```python
from build123d import *
from OCP.BRepFilletAPI import BRepFilletAPI_MakeChamfer

# Parameters (mm, degrees)
BOSS_EXTRUDE1_DEPTH     = 2.4
CUT_EXTRUDE1_DEPTH      = 15.66535032
CUT_EXTRUDE1_DEPTH_BACK = 2.1
SKETCH4_R               = 0.55
CUT_EXTRUDE2_START      = -9
CUT_EXTRUDE2_DEPTH      = 9
SKETCH6_W               = 4.2
SKETCH6_H               = 1.75
BOSS_EXTRUDE2_DEPTH     = 0.75
BOSS_EXTRUDE3_DEPTH     = 0.5
FILLET1_R               = 1
FILLET2_R               = 2
FILLET3_R               = 1
FILLET4_R               = 2
FILLET6_R               = 0.5
FILLET8_R               = 0.6
FILLET9_R               = 3
FILLET10_R              = 3
CHAMFER1_SIZE           = 0.3
CHAMFER1_SIZE2          = 0.357526078


# Read off the part's stored shape, not the designer's step: Cut-Extrude2
# Some blends are built 0.0001 mm under size
with BuildPart() as part:
    # Sketch1 → Boss-Extrude1 (new body)
    with BuildSketch(Plane(origin=(0, 0, 0), x_dir=(1, 0, 0), z_dir=(0, 1, 0))):
        Polygon((-2.1, 0), (-2.1, 5.75), (-1.1, 5.75), (-1.1, 7.25), (-2.1, 7.25), (-4.1, 7.25), (-4.1, 1), (-6.55, -1), (-6.55, -5.65), (-4.05, -5.65), (-4.05, -1.75), (4.05, -1.75), (4.05, -5.65), (6.55, -5.65), (6.55, -1), (4.1, 1), (4.1, 7.25), (2.1, 7.25), (1.1, 7.25), (1.1, 5.75), (2.1, 5.75), (2.1, 0), align=None)
    extrude(amount=BOSS_EXTRUDE1_DEPTH)

    # Sketch4 → Cut-Extrude1 (cut, two sides: drawn at the far end of the back side and taken through both)
    with BuildSketch(Plane.XY.offset(5.65).offset(-CUT_EXTRUDE1_DEPTH_BACK)):
        with Locations((-5.3, 1.2)):
            Circle(SKETCH4_R)
        with Locations(Location((5.3, 1.2, 0), (0, 0, 180))):
            Circle(SKETCH4_R)
    extrude(amount=CUT_EXTRUDE1_DEPTH + CUT_EXTRUDE1_DEPTH_BACK, mode=Mode.SUBTRACT)

    # Cut-Extrude2 outline → Cut-Extrude2 (cut)
    with BuildSketch(Plane.XY.offset(1.75).offset(CUT_EXTRUDE2_START)):
        Polygon((-1.700147862, 2.4), (0, 0.699852138), (1.700147862, 2.4), align=None)
    extrude(amount=CUT_EXTRUDE2_DEPTH, mode=Mode.SUBTRACT)

    # Sketch6 → Boss-Extrude2 (add)
    with BuildSketch(Plane.XZ):
        with Locations((0, 0.875)):
            Rectangle(SKETCH6_W, SKETCH6_H)
    extrude(amount=BOSS_EXTRUDE2_DEPTH)

    # Sketch7 → Boss-Extrude3 (add)
    with BuildSketch(Plane.XZ):
        Polygon((-2.1, -5.75), (-1.1, -5.75), (-1.1, -7.25), (-4.1, -7.25), (-4.1, -2), (-2.1, -2), align=None)
        Polygon((4.1, -2), (2.1, -2), (2.1, -5.75), (1.1, -5.75), (1.1, -7.25), (4.1, -7.25), align=None)
    extrude(amount=BOSS_EXTRUDE3_DEPTH)

    # Fillet1
    # the kernel refuses this fillet: 1 mm, written as the material it adds along each edge
    with BuildSketch(Plane(origin=(-2.1, 0, 1.75), x_dir=(-1, 0, 0), z_dir=(0, 0, -1))) as fillet1_piece_1:
        with BuildLine():
            CenterArc((0.968245837, -1), FILLET1_R, 90, 75.522487814)
            Line((0, -0.75), (0, 0))
            Line((0, 0), (0.968245837, 0))
        make_face()
    extrude(amount=1.75)
    with BuildSketch(Plane(origin=(2.1, 0, 0), x_dir=(0, -1, 0), z_dir=(0, 0, 1))) as fillet1_piece_2:
        with BuildLine():
            CenterArc((1, 0.968245837), FILLET1_R, 180, 75.522487814)
            Line((0, 0.968245837), (0, 0))
            Line((0, 0), (0.75, 0))
        make_face()
    extrude(amount=1.75)

    # Fillet2
    fillet2_edges = [part.edges().sort_by_distance(p)[0] for p in [
        (-2.1, -0.75, 0.875),
        (2.1, -0.75, 0.875),
    ]]
    fillet(fillet2_edges, radius=FILLET2_R)

    # Fillet3
    fillet3_edges = [part.edges().sort_by_distance(p)[0] for p in [
        (-2.1, 0.95, -5.75),
        (2.1, 0.95, -5.75),
        (-2.1, 1.2, 0),
        (2.1, 1.2, 0),
    ]]
    fillet(fillet3_edges, radius=FILLET3_R - 0.0001)  # a hair under: the kernel refuses the full size

    # Fillet4
    fillet4_edges = [part.edges().sort_by_distance(p)[0] for p in [
        (-4.1, 0.95, -7.25),
        (4.1, 0.95, -7.25),
    ]]
    fillet(fillet4_edges, radius=FILLET4_R)

    # Fillet6
    fillet6_edges = [part.edges().sort_by_distance(p)[0] for p in [
        (-1.1, 0.649926069, -7.25),
        (1.1, 0.649926069, -7.25),
    ]]
    fillet(fillet6_edges, radius=FILLET6_R)

    # Fillet8
    fillet8_edges = [part.edges().sort_by_distance(p)[0] for p in [
        (-4.05, 1.2, 1.75),
        (4.05, 1.2, 1.75),
    ]]
    fillet(fillet8_edges, radius=FILLET8_R)

    # Fillet9
    fillet9_edges = [part.edges().sort_by_distance(p)[0] for p in [
        (-6.55, 1.2, 1),
        (6.55, 1.2, 1),
    ]]
    fillet(fillet9_edges, radius=FILLET9_R)

    # Fillet10
    fillet10_edges = [part.edges().sort_by_distance(p)[0] for p in [
        (-4.1, 1.2, -1),
        (4.1, 1.2, -1),
    ]]
    fillet(fillet10_edges, radius=FILLET10_R)

    # Chamfer1: one chamfer whose edges measure the first distance from different faces: ONE call of the kernel's chamfer builder (chamfer() names one face for all edges)
    chamfer1_edges_1 = [part.edges().sort_by_distance(p)[0] for p in [
        (5.3, 2.4, 5.65),
    ]]
    chamfer1_side_1 = [part.faces().sort_by_distance(p)[0] for p in [
        (3.921880383, 2.4, -0.274216986),
    ]]
    chamfer1_edges_2 = [part.edges().sort_by_distance(p)[0] for p in [
        (-5.3, 2.4, 5.65),
    ]]
    chamfer1_side_2 = [part.faces().sort_by_distance(p)[0] for p in [
        (-3.921880383, 2.4, -0.274216986),
    ]]
    chamfer1 = BRepFilletAPI_MakeChamfer(part.part.solid().wrapped)
    for e in chamfer1_edges_1:
        chamfer1.Add(CHAMFER1_SIZE, CHAMFER1_SIZE2, e.wrapped, chamfer1_side_1[0].wrapped)  # the first distance lies on this face
    for e in chamfer1_edges_2:
        chamfer1.Add(CHAMFER1_SIZE, CHAMFER1_SIZE2, e.wrapped, chamfer1_side_2[0].wrapped)  # the first distance lies on this face
    add(Compound.cast(chamfer1.Shape()), mode=Mode.REPLACE)


solid = part.part
```
Here's how the part is built. I have some questions about the finished solid (model axes, mm). A direction names the side the tool comes from. Give positions to 0.01 mm unless a question says otherwise; leave off trailing zeros. Loops run counter-clockwise (first coordinate to the right, second up) from the corner with the lowest first, then second, coordinate; pieces in that order, holes last. Notation, with made-up numbers: M 10,36.25 L 55,36.25 A25 ccw 55,62.25 Z; hole C 39,70.5 d8. An arc over 180 degrees is marked long. Use one line per item in the form item = value. Start each with the question number.
Q1. Thinking about a two-plate mould opening in X: for faces 1 (the cylindrical face through (1.799, 1.217, -0.285)), 2 (the flat face through (4, 2.4, -1)), 3 (the cylindrical face through (-1.782, -0.624, 0.887)), which applies, +X half, -X half, draft (parallel to the pull), parting line (faces both ways), or undercut?
Q2. Will these pins go through, and if not, where does the flat tip stop? pin 1 Ø0.8 at (y, z) = (1, -4) entering from -X; pin 2 Ø1.5 at (x, y) = (1.5, 2) entering from +Z; pin 3 Ø1.4 at (y, z) = (1.5, -4) entering from +X.
Q3. Which directions (+Z, -Z, +X, -X, +Y, -Y) give clear straight access to the entire face, cutting with the end or side of a thin tool? Please do faces 4 (the flat face through (4.05, 1, 4)), 5 (the flat face through (-5, 1, 3.55)), 6 (the flat face through (3, -0.5, -5)), 7 (the cylindrical face through (-1.799, 1.217, -0.285)), 8 (the flat face through (0.8, 1.5, 0.8)).
Q4. If we section it at A-A (z = 3): Write out the boundary of the cut face in (x, y).
Q5. If we section it at B-B (z = -4): Write out the boundary of the cut face in (x, y), then the cut area to 3 significant figures.
Q6. If we section it at C-C (z = 1): Write out the boundary of the cut face in (x, y).
Q7. I need wall thicknesses on line 1 along X through (y, z) = (1.2, 4.25); line 2 along Y through (x, z) = (-5.3, 4.2); line 3 along X through (y, z) = (1.1, -4.25). Which ranges of each line are inside material? Lowest first, please.
Taken from the geometry:
q1.face_1 = undercut
q1.face_2 = draft
q1.face_3 = -X half
q2.pin_1 = -4.1
q2.pin_2 = 1.75
q2.pin_3 = 4.1
q3.face_4 = +Z, +Y, -Y
q3.face_5 = +Z
q3.face_6 = -Z, +X, -X, -Y
q3.face_7 = +Y, -Y
q3.face_8 = +Z, -Z, +Y
q4.outline = M -6.55,0 L -4.05,0 L -4.05,2.4 L -6.55,2.4 Z; M 4.05,0 L 6.55,0 L 6.55,2.4 L 4.05,2.4 Z
q5.outline = M -4.1,-0.5 L -2.1,-0.5 L -2.1,2.4 L -4.1,2.4 Z; M 2.1,-0.5 L 4.1,-0.5 L 4.1,2.4 L 2.1,2.4 Z
q5.area = 11.6 mm^2
q6.outline = M -6.19,0 L -3.07,0 A1 cw -2.41,-0.25 A2 ccw -1.08,-0.75 L 1.08,-0.75 A2 ccw 2.41,-0.25 A1 cw 3.07,0 L 6.19,0 L 6.19,2.4 L 1.7,2.4 L 0,0.7 L -1.7,2.4 L -6.19,2.4 Z
q7.line_1 = -6.55 to -5.85, -4.75 to -4.05, 4.05 to 4.75, 5.85 to 6.55
q7.line_2 = 0 to 0.65, 1.75 to 2.4
q7.line_3 = -4.1 to -2.1, 2.1 to 4.1
